from build123d import *

# Parameters (mm, degrees)
F1_DEPTH = 19.05
F2_DEPTH = 12.7
F3_R     = 5.07999


# Not quite as in the source:
# - a fillet or chamfer is up to 0.001 mm smaller than in the source, because OpenCascade refuses the exact size


with BuildPart() as f1:
    # F0 (on Front) → F1 (new body, symmetric)
    with BuildSketch(Plane.XZ):
        Polygon((-8.1223546189, -57.6977613127), (-8.1223546189, 12.1522386873), (7.1176453811, 12.1522386873), (7.1176453811, -57.6977613127), (12.1976453811, -57.6977613127), (12.1976453811, -16.6773311794), (12.1976453811, -5.3586508704), (12.1976453811, 3.81), (12.1976453811, 9.9853777035), (12.1976453811, 18.5022386873), (-13.2023546189, 18.5022386873), (-13.2023546189, -57.6977613127), align=None)
    extrude(amount=F1_DEPTH, both=True)

    # F0 (on Front) → F2 (join, symmetric)
    with BuildSketch(Plane.XZ):
        Polygon((20.4923357815, 3.81), (12.1976453811, 9.9853777035), (12.1976453811, 3.81), (16.9246122241, 3.81), align=None)
        Polygon((12.1976453811, -5.3586508704), (12.1976453811, -16.6773311794), (19.8778546898, 0), (16.9246122241, 0), align=None)
        with BuildLine():
            Line((16.9246122241, 0), (19.8778546898, 0))
            ThreePointArc((19.8778546898, 0), (18.401233457, 1.2428820016), (16.9246122241, 0))
        make_face()
    extrude(amount=F2_DEPTH, both=True)

    # F3 (radius 5.08 in the source; OpenCascade refuses exactly that, so slightly less here)
    f3_edges = [f1.edges().sort_by_distance(p)[0] for p in [
        (12.197645, 0, 18.502239),
        (-13.202355, 0, 18.502239),
        (-0.502355, -19.05, 18.502239),
        (-0.502355, 19.05, 18.502239),
        (7.117645, 0, -57.697761),
        (-8.122355, 0, -57.697761),
    ]]
    fillet(f3_edges, radius=F3_R)


solid = f1.part
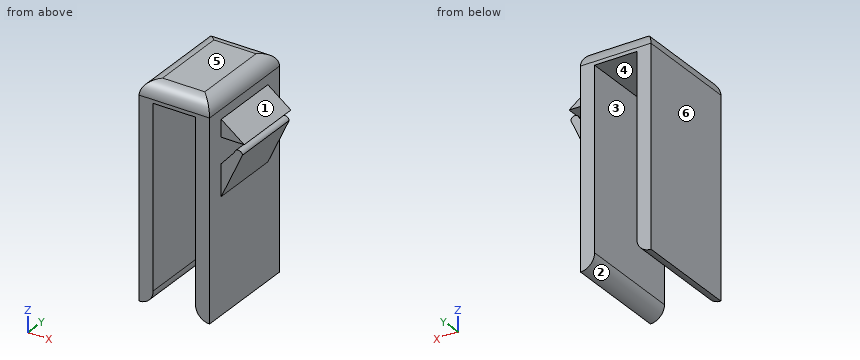
Can you work these out from the model? Positions are in its coordinate system, mm. Face numbers are marked on the shaded views. A direction names the side the tool comes from. Coordinates: 2 decimals unless noted, no trailing zeros. Write each loop counter-clockwise with the first axis right and the second up, starting at its lowest first coordinate (ties: lowest second). Pieces come first, ordered by that corner, then holes. Notation, with made-up numbers: (36, 13) -> (47, 13) arc R30 cw to (47, 50) -> close; hole circle Ø2 at (75, 38). An arc over 180 degrees is marked (long way). Write item = value, one per line.
(1) Imagine slicing it at A-A (z = -34). Please give me the cut outline in (x, y), and give its area (3 significant figures).
Verdict:
outline = (-13.2, -19.05) -> (-8.12, -19.05) -> (-8.12, 19.05) -> (-13.2, 19.05) -> close; (7.12, -19.05) -> (12.2, -19.05) -> (12.2, 19.05) -> (7.12, 19.05) -> close
area = 387 mm^2
(2) For pin 1 (10 mm diameter, centred on y = 12.5, z = -9.5, fed in from +X); pin 2 (3 mm diameter, centred on y = 10.5, z = -19, fed in from +X); pin 3 (8.5 mm diameter, centred on x = 17, z = -11.5, fed in from +Y), each with a flat end and sliding along its axis, tell me the tip position at first contact or that it passes through.
Verdict:
pin_1 = 17.81
pin_2 = 12.2
pin_3 = 12.7
(3) Thinking about a two-plate mould opening in X: for the marked faces 3, 4, 5 and 6, which applies, +X half, -X half, draft (parallel to the pull), parting line (faces both ways), or undercut?
Verdict:
face_3 = undercut
face_4 = undercut
face_5 = draft
face_6 = -X half
(4) Imagine slicing it at D-D (x = 5). Please give me the cut outline in (y, z).
Verdict:
outline = (-19.05, 12.15) -> (19.05, 12.15) -> (19.05, 13.42) arc R5.08 ccw to (13.97, 18.5) -> (-13.97, 18.5) arc R5.08 ccw to (-19.05, 13.42) -> close
(5) Imagine slicing it at B-B (x = 13). Please give me the cut outline in (y, z), and give its area (3 significant figures).
Verdict:
outline = (-12.7, -14.94) -> (12.7, -14.94) -> (12.7, -4.45) -> (-12.7, -4.45) -> close; (-12.7, 3.81) -> (12.7, 3.81) -> (12.7, 9.39) -> (-12.7, 9.39) -> close
area = 408 mm^2
(6) If I drill on probe 1 along X at (y, z) = (3.5, -33); probe 2 along X at (y, z) = (-12, -4); probe 3 along X at (y, z) = (-10, -9), over which ranges is the centre line in solid material (lowest first)?
Verdict:
probe_1 = -13.2 to -8.12, 7.12 to 12.2
probe_2 = -13.2 to -8.12, 7.12 to 12.2, 13.4 to 18.04
probe_3 = -13.2 to -8.12, 7.12 to 15.73
(7) On a 3-axis mill with a long thin cutter (end or side, diameter ignored), from which of +Z, -Z, +X, -X, +Y, -Y can I reach the whole of each face in a straight line? I mean the marked faces 1 and 2. Say none if no direction works.
Verdict:
face_1 = +Z, +X, +Y, -Y
face_2 = -Z, +Y, -Y
